```python
from build123d import *

# Parameters (mm, degrees)
SKETCH_R   = 4
SKETCH_R_2 = 3
PAD_DEPTH  = 10


with BuildPart() as part:
    # Sketch → Pad (new body)
    with BuildSketch(Plane.XY):
        with BuildLine():
            Line((-19.818265, 2.465513), (-10, 6.314027))
            Line((-10, 6.314027), (-10, 14))
            Line((-10, 14), (10, 14))
            Line((10, 14), (10, 6.314027))
            Line((10, 6.314027), (19.818265, 2.465513))
            ThreePointArc((19.863348, -2.447363), (21.499889, 0.0243), (19.818265, 2.465513))
            Line((19.863348, -2.447363), (3.058498, -9.392862))
            ThreePointArc((-3.058498, -9.392862), (0, -10), (3.058498, -9.392862))
            Line((-3.058498, -9.392862), (-19.863348, -2.447363))
            ThreePointArc((-19.818265, 2.465513), (-21.499889, 0.0243), (-19.863348, -2.447363))
        make_face()
        Circle(SKETCH_R, mode=Mode.SUBTRACT)
        with Locations((-16.25, 0)):
            Circle(SKETCH_R_2, mode=Mode.SUBTRACT)
        with Locations((16.25, 0)):
            Circle(SKETCH_R_2, mode=Mode.SUBTRACT)
    extrude(amount=PAD_DEPTH)


solid = part.part
```
Model file for the job. Use its own axes, mm. A direction names the side the tool comes from. Give positions to 0.01 mm unless a question says otherwise; leave off trailing zeros. Write each loop counter-clockwise with the first axis right and the second up, starting at its lowest first coordinate (ties: lowest second). Pieces come first, ordered by that corner, then holes. Notation, with made-up numbers: (80.5, 0) - (107.5, 0) arc R16 ccw to (107.5, 19) - close; hole circle Ø4 at (-7, -16.5). An arc over 180 degrees is marked (long way). One line per question, with ' | ' between items. Start each with the question number.
(1) Pin check, flat tips, straight feed: P1, Ø4, axis at x = 6.5, z = 6.5, coming from the -Y side; P2, Ø4, axis at y = 9, z = 7, coming from the +X side; P3, Ø2, axis at x = 12.5, z = 2, coming from the +Y side. Stop position of each tip, or through.
(2) Slice it at C-C on x = -15. Write the cut outline in (y, z), plus the area to 3 significant figures.
(3) Slice it at B-B on y = 0. Write the cut outline in (x, z).
(4) Slice it at A-A on z = 6. Write the cut outline in (x, y).
(5) Two-plate mould, pull along Y, no slides. Class faces 3 (the face through (-14.98, 4.36, 4.93)), 4 (the face through (-0.867, -3.905, 4.93)), 5 (the face through (10, 10, 5)), 6 (the face through (11.58, -5.87, 4.93)): +Y half, -Y half, draft (parallel to the pull), parting line (faces both ways), or undercut.
(6) Wall check: line 1 along Y through (x, z) = (0, 3.5); line 2 along Y through (x, z) = (16.5, 8); line 3 along X through (y, z) = (9.75, 8.25). Give the ranges that are in metal, low to high. Write a range as from..to.
(7) 3-axis set-ups, long thin cutter, end or side, ignore diameter. For faces 1 (the face through (-11.34, -5.97, 4.93)), 2 (the face through (-10, 10, 5)): which of +Z, -Z, +X, -X, +Y, -Y reach the whole face in a straight line?
(8) Slice it at D-D on y = 11. Write the cut outline in (x, z).
Results below:
1) P1: y = -8.8 | P2: x = 10 | P3: y = 5.73
2) outline: (-4.46, 0) - (-2.73, 0) - (-2.73, 10) - (-4.46, 10) - close; (2.73, 0) - (4.35, 0) - (4.35, 10) - (2.73, 10) - close | area: 33.6 mm^2
3) outline: (-21.5, 0) - (-19.25, 0) - (-19.25, 10) - (-21.5, 10) - close; (-13.25, 0) - (-4, 0) - (-4, 10) - (-13.25, 10) - close; (4, 0) - (13.25, 0) - (13.25, 10) - (4, 10) - close; (19.25, 0) - (21.5, 0) - (21.5, 10) - (19.25, 10) - close
4) outline: (-19.86, -2.45) - (-3.06, -9.39) arc R8.01 ccw to (3.06, -9.39) - (19.86, -2.45) arc R2.65 ccw to (19.82, 2.47) - (10, 6.31) - (10, 14) - (-10, 14) - (-10, 6.31) - (-19.82, 2.47) arc R2.65 ccw to start; hole circle Ø6 at (-16.25, 0); hole circle Ø8 at (0, 0); hole circle Ø6 at (16.25, 0)
5) face 3: +Y half | face 4: undercut | face 5: draft | face 6: -Y half
6) line 1: -10..-4, 4..14 | line 2: -3.84..-2.99, 2.99..3.77 | line 3: -10..10
7) face 1: +Z, -Z, -X, -Y | face 2: +Z, -Z, -X, +Y
8) outline: (-10, 0) - (10, 0) - (10, 10) - (-10, 10) - close
